The listing builds one solid part. Answer for the finished solid, in the listing's coordinates (mm). A direction names the side the tool comes from. Round coordinates to 2 decimals unless told otherwise and drop trailing zeros. Loops run counter-clockwise (first coordinate to the right, second up) from the corner with the lowest first, then second, coordinate; pieces in that order, holes last. Notation, with made-up numbers: (-28, -33.75) -> (24, -33.75) arc R18 cw to (24, -27.75) -> close; hole circle Ø4 at (39.5, -5). An arc over 180 degrees is marked (long way). Answer in a Markdown table with one row per item. Add a question column.
```python
from build123d import *

# Parameters (mm, degrees)
SKETCH1_W           = 75
SKETCH1_H           = 10
BOSS_EXTRUDE5_DEPTH = 25
BOSS_EXTRUDE6_DEPTH = 15
BOSS_EXTRUDE7_DEPTH = 5
FILLET2_R           = 1
FILLET3_R           = 1


with BuildPart() as part:
    # Sketch1 → Boss-Extrude5 (new, symmetric)
    with BuildSketch(Plane.XY):
        with Locations((0, 5)):
            Rectangle(SKETCH1_W, SKETCH1_H)
    extrude(amount=BOSS_EXTRUDE5_DEPTH, both=True)

    # Sketch1<9> → Boss-Extrude6 (add, symmetric)
    with BuildSketch(Plane.XY):
        with BuildLine():
            Line((-5, 20.635083269), (-5, 10))
            Line((-5, 10), (5, 10))
            Line((5, 10), (5, 20.635083269))
            ThreePointArc((5, 20.635083269), (15.811388301, 27.752551286), (20, 40))
            Line((20, 40), (12, 40))
            ThreePointArc((12, 40), (0, 28), (-12, 40))
            Line((-12, 40), (-20, 40))
            ThreePointArc((-20, 40), (-15.811388301, 27.752551286), (-5, 20.635083269))
        make_face()
    extrude(amount=BOSS_EXTRUDE6_DEPTH, both=True)

    # Sketch1<10> → Boss-Extrude7 (add, symmetric)
    with BuildSketch(Plane.XY):
        with BuildLine():
            Line((5, 10), (37.5, 10))
            Line((37.5, 10), (20, 40))
            ThreePointArc((20, 40), (15.811388301, 27.752551286), (5, 20.635083269))
            Line((5, 20.635083269), (5, 10))
        make_face()
        with BuildLine():
            Line((-20, 40), (-37.5, 10))
            Line((-37.5, 10), (-5, 10))
            Line((-5, 10), (-5, 20.635083269))
            ThreePointArc((-5, 20.635083269), (-15.811388301, 27.752551286), (-20, 40))
        make_face()
    extrude(amount=BOSS_EXTRUDE7_DEPTH, both=True)

    # Fillet2
    fillet2_edges = [part.edges().sort_by_distance(p)[0] for p in [
        (-12, 40, 0),
        (-15.811388301, 27.752551286, -15),
        (-5, 15.317541634, -15),
        (5, 15.317541634, 15),
        (15.811388301, 27.752551286, -15),
        (0, 28, 15),
        (12, 40, 0),
        (-15.811388301, 27.752551286, 15),
        (-5, 15.317541634, 15),
        (15.811388301, 27.752551286, 15),
        (0, 28, -15),
        (5, 15.317541634, -15),
    ]]
    fillet(fillet2_edges, radius=FILLET2_R)

    # Fillet3
    # the kernel refuses this fillet: 1 mm, written as the material it adds along each edge
    with BuildSketch(Plane(origin=(5, 10, -14), x_dir=(1, 0, 0), z_dir=(0, 0, 1)), Plane(origin=(5, 10, 2.5), x_dir=(1, 0, 0), z_dir=(0, 0, 1))) as fillet3_piece_1:
        with BuildLine():
            CenterArc((FILLET3_R, FILLET3_R), FILLET3_R, 180, 90)
            Line((0, FILLET3_R), (0, 0))
            Line((0, 0), (FILLET3_R, 0))
        make_face()
    extrude(amount=11.5)
    with BuildSketch(Plane(origin=(-5, 10, -14), x_dir=(-1, 0, 0), z_dir=(0, 0, 1)), Plane(origin=(-5, 10, 2.5), x_dir=(-1, 0, 0), z_dir=(0, 0, 1))) as fillet3_piece_2:
        with BuildLine():
            CenterArc((FILLET3_R, -FILLET3_R), FILLET3_R, 90, 90)
            Line((0, -FILLET3_R), (0, 0))
            Line((0, 0), (FILLET3_R, 0))
        make_face()
    extrude(amount=11.5)
    with BuildSketch(Plane(origin=(2.5, 10, 5), x_dir=(0, 0, 1), z_dir=(1, 0, 0))) as fillet3_piece_3_section:
        with BuildLine():
            CenterArc((FILLET3_R, -FILLET3_R), FILLET3_R, 90, 90)
            Line((0, -FILLET3_R), (0, 0))
            Line((0, 0), (FILLET3_R, 0))
        make_face()
    fillet3_piece_3 = extrude(amount=35, mode=Mode.PRIVATE)
    fillet3_piece_3 = split(fillet3_piece_3, bisect_by=Plane(origin=(28.832812489, 24.858035733, 5.226395114), z_dir=(-0.8637789008984333, -0.5038710255240864, 0)), keep=Keep.TOP, mode=Mode.PRIVATE)
    add(fillet3_piece_3)
    with BuildSketch(Plane(origin=(2.5, 10, -5), x_dir=(0, 0, -1), z_dir=(1, 0, 0))) as fillet3_piece_4_section:
        with BuildLine():
            CenterArc((FILLET3_R, FILLET3_R), FILLET3_R, 180, 90)
            Line((0, FILLET3_R), (0, 0))
            Line((0, 0), (FILLET3_R, 0))
        make_face()
    fillet3_piece_4 = extrude(amount=35, mode=Mode.PRIVATE)
    fillet3_piece_4 = split(fillet3_piece_4, bisect_by=Plane(origin=(28.832812489, 24.858035733, -5.226395114), z_dir=(-0.8637789008984333, -0.5038710255240864, 0)), keep=Keep.TOP, mode=Mode.PRIVATE)
    add(fillet3_piece_4)
    with BuildSketch(Plane(origin=(-37.5, 10, 5), x_dir=(0, 0, 1), z_dir=(1, 0, 0))) as fillet3_piece_5_section:
        with BuildLine():
            CenterArc((FILLET3_R, -FILLET3_R), FILLET3_R, 90, 90)
            Line((0, -FILLET3_R), (0, 0))
            Line((0, 0), (FILLET3_R, 0))
        make_face()
    fillet3_piece_5 = extrude(amount=35, mode=Mode.PRIVATE)
    fillet3_piece_5 = split(fillet3_piece_5, bisect_by=Plane(origin=(-33.259418432, 17.269568402, 5.226886144), z_dir=(0.8637789008984326, -0.5038710255240878, 0)), keep=Keep.TOP, mode=Mode.PRIVATE)
    add(fillet3_piece_5)
    with BuildSketch(Plane(origin=(-37.5, 10, -5), x_dir=(0, 0, -1), z_dir=(1, 0, 0))) as fillet3_piece_6_section:
        with BuildLine():
            CenterArc((FILLET3_R, FILLET3_R), FILLET3_R, 180, 90)
            Line((0, FILLET3_R), (0, 0))
            Line((0, 0), (FILLET3_R, 0))
        make_face()
    fillet3_piece_6 = extrude(amount=35, mode=Mode.PRIVATE)
    fillet3_piece_6 = split(fillet3_piece_6, bisect_by=Plane(origin=(-33.259418432, 17.269568402, -5.226886144), z_dir=(0.8637789008984326, -0.5038710255240878, 0)), keep=Keep.TOP, mode=Mode.PRIVATE)
    add(fillet3_piece_6)
    with BuildSketch(Plane(origin=(-4, 10, 15), x_dir=(0, 0, 1), z_dir=(1, 0, 0))) as fillet3_piece_7:
        with BuildLine():
            CenterArc((FILLET3_R, -FILLET3_R), FILLET3_R, 90, 90)
            Line((0, -FILLET3_R), (0, 0))
            Line((0, 0), (FILLET3_R, 0))
        make_face()
    extrude(amount=8)
    with BuildSketch(Plane(origin=(-4, 10, -15), x_dir=(0, 0, -1), z_dir=(1, 0, 0))) as fillet3_piece_8:
        with BuildLine():
            CenterArc((FILLET3_R, FILLET3_R), FILLET3_R, 180, 90)
            Line((0, FILLET3_R), (0, 0))
            Line((0, 0), (FILLET3_R, 0))
        make_face()
    extrude(amount=8)
    with BuildSketch(Plane(origin=(-4, 10, 14), x_dir=(0, 0, 1), z_dir=(1, 0, 0))) as fillet3_piece_9:
        with BuildLine():
            CenterArc((1 + FILLET3_R, -FILLET3_R), FILLET3_R, 90, 90)
            Line((1, -FILLET3_R), (1, 0))
            Line((1, 0), (1 + FILLET3_R, 0))
        make_face()
    revolve(axis=Axis((-4, 10, 14), (0, -1, 0)), revolution_arc=90)
    with BuildSketch(Plane(origin=(4, 10, 14), x_dir=(1, 0, 0), z_dir=(0, 0, -1))) as fillet3_piece_10:
        with BuildLine():
            CenterArc((1 + FILLET3_R, -FILLET3_R), FILLET3_R, 90, 90)
            Line((1, -FILLET3_R), (1, 0))
            Line((1, 0), (1 + FILLET3_R, 0))
        make_face()
    revolve(axis=Axis((4, 10, 14), (0, -1, 0)), revolution_arc=90)
    with BuildSketch(Plane(origin=(4, 10, -14), x_dir=(0, 0, -1), z_dir=(-1, 0, 0))) as fillet3_piece_11:
        with BuildLine():
            CenterArc((1 + FILLET3_R, -FILLET3_R), FILLET3_R, 90, 90)
            Line((1, -FILLET3_R), (1, 0))
            Line((1, 0), (1 + FILLET3_R, 0))
        make_face()
    revolve(axis=Axis((4, 10, -14), (0, -1, 0)), revolution_arc=90)
    with BuildSketch(Plane(origin=(-4, 10, -14), x_dir=(-1, 0, 0), z_dir=(0, 0, 1))) as fillet3_piece_12:
        with BuildLine():
            CenterArc((1 + FILLET3_R, -FILLET3_R), FILLET3_R, 90, 90)
            Line((1, -FILLET3_R), (1, 0))
            Line((1, 0), (1 + FILLET3_R, 0))
        make_face()
    revolve(axis=Axis((-4, 10, -14), (0, -1, 0)), revolution_arc=90)


solid = part.part
```
Item 1: Consider L1, parallel to Y at x = -10.5, z = -9.5; L2, parallel to Y at x = -24, z = 7.5; L3, parallel to X at y = 37, z = -6.5. Determine where each line is inside the solid, lowest interval first. Write a range as from..to.
Item 2: Section C-C, the plane x = 28 is taken. Write down the section's boundary in (y, z).
Item 3: Section A-A, the plane z = -0.5 is taken. Write down the section's boundary in (x, y), and give its area (3 significant figures).
Item 4: Section D-D, the plane z = 11 is taken. Write down the section's boundary in (x, y), and give its area (3 significant figures).
Item 5: Flat-ended cylindrical pins translate along their axes: P1, Ø3, axis at x = -28, y = 32.5, coming from the -Z side; P2, Ø1.5, axis at x = 15.5, y = 14.5, coming from the -Z side; P3, Ø23, axis at x = -18.5, y = 28.5, coming from the +Z side; P4, Ø8.5, axis at x = 17, y = 20, coming from the +Z side. Find the tip coordinate at first contact, or state that the pin passes through.
Item 6: For faces 5 (the flat face through (-1, 10, -17)), 6 (the flat face through (5, 16, -9)), 7 (the cylindrical face through (16, 28, 10)), determine the directions among +Z, -Z, +X, -X, +Y, -Y from which every point of the face is accessible in a straight line to the end or side of a thin tool.
Item 7: The mould has two halves that part along Y. Classify faces 1 (the flat face through (-5, 16, -9)), 2 (the flat face through (-1, 0, 0)), 3 (the flat face through (17, 40, 0)), 4 (the flat face through (21, 19, 5)): +Y half, -Y half, draft (parallel to the pull), parting line (faces both ways), or undercut.
Item 8: Section B-B, the plane y = 16 is taken. Write down the section's boundary in (x, z).
Here are the results:
| question | item | result |
|---|---|---|
| 1 | L1 | y = 0..10, 22.98..34.19 |
| 1 | L2 | y = 0..10 |
| 1 | L3 | x = -19.77..-11.62, 11.62..19.77 |
| 2 | outline | (0, -25) -> (10, -25) -> (10, -6) arc R1 cw to (11, -5) -> (26.29, -5) -> (26.29, 5) -> (11, 5) arc R1 cw to (10, 6) -> (10, 25) -> (0, 25) -> close |
| 3 | outline | (-37.5, 0) -> (37.5, 0) -> (37.5, 10) -> (20, 40) -> (12.96, 40) arc R1 ccw to (11.96, 39.08) arc R12 cw to (-11.96, 39.08) arc R1 ccw to (-12.96, 40) -> (-20, 40) -> (-37.5, 10) -> close |
| 3 | area | 2,250 mm² |
| 4 | outline | (-37.5, 0) -> (37.5, 0) -> (37.5, 10) -> (6, 10) arc R1 cw to (5, 11) -> (5, 20.64) arc R20 ccw to (20, 40) -> (12.96, 40) arc R1 ccw to (11.96, 39.08) arc R12 cw to (-11.96, 39.08) arc R1 ccw to (-12.96, 40) -> (-20, 40) arc R20 ccw to (-5, 20.64) -> (-5, 11) arc R1 cw to (-6, 10) -> (-37.5, 10) -> close |
| 4 | area | 1,250 mm² |
| 5 | P1 | passes through |
| 5 | P2 | stops at z = -5 |
| 5 | P3 | stops at z = 15 |
| 5 | P4 | stops at z = 5 |
| 6 | face 5 | -Z |
| 6 | face 6 | -Z, +X |
| 6 | face 7 | +Z, +X |
| 7 | face 1 | undercut |
| 7 | face 2 | -Y half |
| 7 | face 3 | +Y half |
| 7 | face 4 | undercut |
| 8 | outline | (-34, -5) -> (-5, -5) -> (-5, -14) arc R1 ccw to (-4, -15) -> (4, -15) arc R1 ccw to (5, -14) -> (5, -5) -> (34, -5) -> (34, 5) -> (5, 5) -> (5, 14) arc R1 ccw to (4, 15) -> (-4, 15) arc R1 ccw to (-5, 14) -> (-5, 5) -> (-34, 5) -> close |
